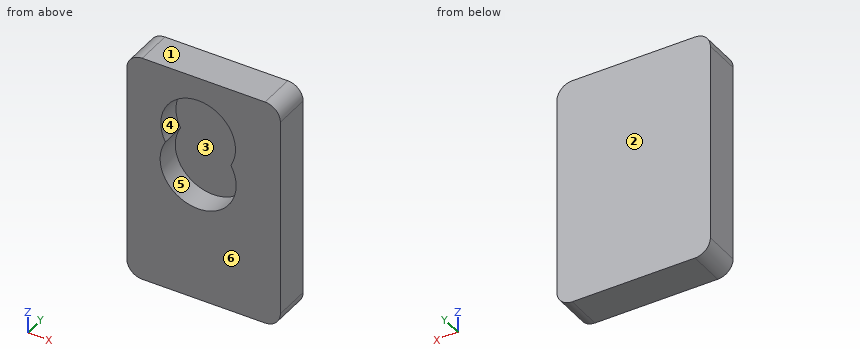
from build123d import *

# Parameters (mm, degrees)
F0_W     = 50
F0_H     = 75
F1_DEPTH = 12
F3_DEPTH = 8
F4_R     = 5


with BuildPart() as f1:
    # F0 (on Front) → F1 (new body)
    with BuildSketch(Plane.XZ):
        with Locations((25, 37.5)):
            Rectangle(F0_W, F0_H)
    extrude(amount=F1_DEPTH)

    # F2 (on face) → F3 (cut)
    with BuildSketch(Plane.XZ.offset(12)):
        with BuildLine():
            ThreePointArc((12.545369, 49.367264), (23.213018, 30.672003), (33.880667, 49.367264))
            ThreePointArc((33.880667, 49.367264), (23.213018, 67.418774), (12.545369, 49.367264))
        make_face()
    extrude(amount=-F3_DEPTH, mode=Mode.SUBTRACT)

    # F4
    f4_edges = [f1.edges().sort_by_distance(p)[0] for p in [
        (50, -6, 0),
        (50, -6, 75),
        (0, -6, 75),
        (0, -6, 0),
    ]]
    fillet(f4_edges, radius=F4_R)


solid = f1.part
CAD build for the part. Positions are in the model's coordinates, mm. Face numbers are marked on the shaded views. A direction names the side the tool comes from. Give positions to 0.01 mm unless a question says otherwise; leave off trailing zeros. Order: outer loops, then holes, each group sorted by start corner. A loop starts at its lowest first (then second) coordinate and runs counter-clockwise, first axis right, second up. Notation, with made-up numbers: (-28, -8) - (18, -8) arc R35 cw to (18, 26) - close; hole circle Ø10 at (87.5, 74). An arc over 180 degrees is marked (long way). Answer in a Markdown table with one row per item.
1. Saw through at C-C, the plane z = 54. Give the cut face in (x, y), plus the area to 3 significant figures.
Data:
| item | result |
|---|---|
| outline | (0, -12) - (11.1, -12) - (11.1, -4) - (35.33, -4) - (35.33, -12) - (50, -12) - (50, 0) - (0, 0) - close |
| area | 406 mm² |
2. Saw through at A-A, the plane y = -10.75. Give the cut face in (x, z).
Data:
| item | result |
|---|---|
| outline | (0, 5) arc R5 ccw to (5, 0) - (45, 0) arc R5 ccw to (50, 5) - (50, 70) arc R5 ccw to (45, 75) - (5, 75) arc R5 ccw to (0, 70) - close; hole (12.55, 49.37) arc R12.39 ccw (long way) to (33.88, 49.37) arc R12.18 ccw (long way) to start |
3. Probe probe 1 along X at (y, z) = (-8.25, 43); probe 2 along Y at (x, z) = (30.5, 42.5); probe 3 along Z at (x, y) = (17, -7.25). List the from-to ranges inside material, lowest first. Write a range as [from, to].
Data:
| item | result |
|---|---|
| probe 1 | x = [0, 10.82], [35.6, 50] |
| probe 2 | y = [-4, 0] |
| probe 3 | z = [0, 32.34], [65.71, 75] |
4. Saw through at B-B, the plane x = 33. Give the cut face in (y, z), plus the area to 3 significant figures.
Data:
| item | result |
|---|---|
| outline | (-12, 0) - (0, 0) - (0, 75) - (-12, 75) - (-12, 62.49) - (-4, 62.49) - (-4, 35.46) - (-12, 35.46) - close |
| area | 684 mm² |
5. Flat gauge pins, fed straight in: pin 1 (12.5 mm diameter, centred on x = 17, z = 44.5, fed in from -Y); pin 2 (19.5 mm diameter, centred on x = 23.21, z = 55.24, fed in from -Y). Where does each tip first touch, or does it go through?
Data:
| item | result |
|---|---|
| pin 1 | stops at y = -12 |
| pin 2 | stops at y = -4 |
6. Pull direction Z, two halves, no side cores. Call the marked faces 1, 2, 3 and 4: pulls with the +Z half, pulls with the -Z half, needs draft (parallel to the pull), parting line crosses it, or undercut.
Data:
| item | result |
|---|---|
| face 1 | pulls with the +Z half |
| face 2 | needs draft |
| face 3 | undercut |
| face 4 | undercut |
7. Tool access for the marked faces 5 and 6: list every direction of +Z, -Z, +X, -X, +Y, -Y with a clear straight run to the whole face (end or side of a thin tool).
Data:
| item | result |
|---|---|
| face 5 | -Y |
| face 6 | +Z, -Z, +X, -X, -Y |
